from build123d import *

# Parameters (mm, degrees)
SKETCH1_R           = 3.96875
BOSS_EXTRUDE1_DEPTH = 3.175


with BuildPart() as part:
    # Sketch1 → Boss-Extrude1 (new body)
    with BuildSketch(Plane(origin=(0, 0, 0), x_dir=(1, 0, 0), z_dir=(0, 1, 0))):
        with BuildLine():
            Line((-30.06597498, 6.287799421), (29.93402502, 6.287799421))
            ThreePointArc((29.93402502, 6.287799421), (33.02652847, 5.469090466), (35.308836634, 3.227454594))
            ThreePointArc((35.308836634, 3.227454594), (35.67400594, 2.868792854), (36.168806492, 2.737799421))
            Line((36.168806492, 2.737799421), (39.323343513, 2.737799421))
            ThreePointArc((39.323343513, 2.737799421), (42.023343513, 0.037799421), (39.323343513, -2.662200579))
            Line((39.323343513, -2.662200579), (36.168806492, -2.662200579))
            ThreePointArc((36.168806492, -2.662200579), (35.67400594, -2.793194011), (35.308836634, -3.151855751))
            ThreePointArc((35.308836634, -3.151855751), (33.02652847, -5.393491623), (29.93402502, -6.212200579))
            Line((29.93402502, -6.212200579), (-30.06597498, -6.212200579))
            ThreePointArc((-30.06597498, -6.212200579), (-36.31597498, 0.037799421), (-30.06597498, 6.287799421))
        make_face()
        with Locations(Location((-30.06597498, 0.037799421, 0), (0, 0, 270))):
            Circle(SKETCH1_R, mode=Mode.SUBTRACT)
        with Locations(Location((29.93402502, 0.037799421, 0), (0, 0, 270))):
            Circle(SKETCH1_R, mode=Mode.SUBTRACT)
    extrude(amount=BOSS_EXTRUDE1_DEPTH)


solid = part.part
Can you work these out from the model? Positions are in its coordinate system, mm. A direction names the side the tool comes from. Coordinates: 2 decimals unless noted, no trailing zeros. Loops run counter-clockwise (first coordinate to the right, second up) from the corner with the lowest first, then second, coordinate; pieces in that order, holes last. Notation, with made-up numbers: (88.5, 43) - (109.5, 43) arc R17 cw to (109.5, 68) - close; hole circle Ø2 at (51, -2.5). An arc over 180 degrees is marked (long way). Put each result on its own line as item: value. Start each with the question number.
Item 1: Which directions (+Z, -Z, +X, -X, +Y, -Y) give clear straight access to the entire face, cutting with the end or side of a thin tool? Please do faces 1 (the face through (0, 2, 6.212)), 2 (the face through (38, 2, 2.662)).
Item 2: Suppose I cut it at B-B (x = -29). Please give me the cut outline in (y, z) (3 decimals).
Item 3: For pin 1 (1 mm diameter, centred on y = 0.5, z = 3, fed in from -X); pin 2 (1.6 mm diameter, centred on x = 37, y = 2, fed in from +Z), each with a flat end and sliding along its axis, tell me the tip position at first contact or that it passes through.
Item 4: Suppose I cut it at D-D (x = 29). Please give me the cut outline in (y, z) (3 decimals), and give its area (3 significant figures).
Item 5: Suppose I cut it at C-C (z = 0.5). Please give me the cut outline in (x, y) (3 decimals), and give its area (3 significant figures).
Item 6: If I drill on line 1 along X through (y, z) = (0.85, 0.25); line 2 along X through (y, z) = (0.8, 3); line 3 along Z through (x, y) = (29, 1), over which ranges is the centre line in solid material (lowest first)?
Item 7: Suppose I cut it at A-A (y = 1.25). Please give me the cut outline in (x, z), and give its area (3 significant figures).
Item 8: If we mould it in two halves opening along X, with no side actions, what happens to faces 3 (the face through (32.99, 1.57, -5.49)), 4 (the face through (-26.13, 1.57, -0.55)), 5 (the face through (38, 2, -2.738))? For each: +X half, -X half, draft (parallel to the pull), parting line (faces both ways), or undercut.
Here are the results:
1. face 1: +Z, +X, -X, +Y, -Y
1. face 2: +Z, +X, +Y, -Y
2. outline: (0, -6.288) - (3.175, -6.288) - (3.175, -3.861) - (0, -3.861) - close; (0, 3.785) - (3.175, 3.785) - (3.175, 6.212) - (0, 6.212) - close
3. pin 1: x = -35.78
3. pin 2: z = 2.66
4. outline: (0, -6.288) - (3.175, -6.288) - (3.175, -3.895) - (0, -3.895) - close; (0, 3.819) - (3.175, 3.819) - (3.175, 6.212) - (0, 6.212) - close
4. area: 15.2 mm²
5. outline: (-36.293, 0) - (-33.998, 0) - (-33.998, 3.175) - (-36.293, 3.175) - close; (-26.134, 0) - (26.002, 0) - (26.002, 3.175) - (-26.134, 3.175) - close; (33.866, 0) - (41.969, 0) - (41.969, 3.175) - (33.866, 3.175) - close
5. area: 199 mm²
6. line 1: -36.31 to -34.02, -26.11 to 25.98, 33.89 to 42.01
6. line 2: -35.53 to -32.62, -27.51 to 27.38, 32.49 to 35.42
6. line 3: -6.29 to -3.9, 3.82 to 6.21
7. outline: (-30.07, -6.29) - (29.93, -6.29) arc R6.25 ccw to (35.31, -3.23) arc R1 cw to (36.17, -2.74) - (39.32, -2.74) arc R2.7 ccw to (39.32, 2.66) - (36.17, 2.66) arc R1 cw to (35.31, 3.15) arc R6.25 ccw to (29.93, 6.21) - (-30.07, 6.21) arc R6.25 ccw to start; hole circle Ø7.94 at (-30.07, -0.04); hole circle Ø7.94 at (29.93, -0.04)
7. area: 803 mm²
8. face 3: +X half
8. face 4: undercut
8. face 5: draft
